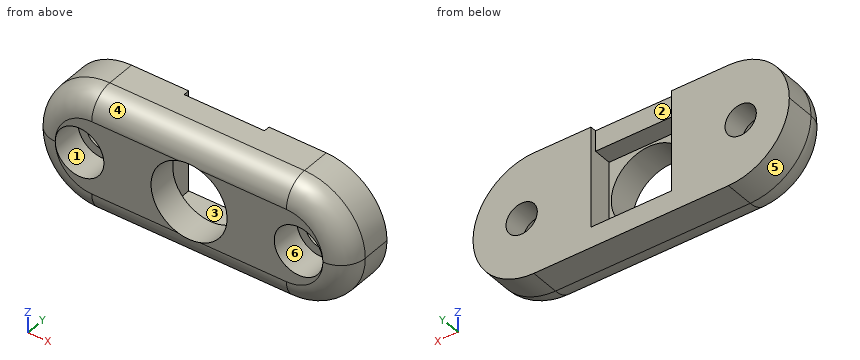
from build123d import *

# Parameters (mm, degrees)
SKETCH1_W                 = 33.02
SKETCH1_H                 = 12.7
SKETCH1_R                 = 3.96875
BOSS_EXTRUDE1_DEPTH       = 5.588
SKETCH2_W                 = 8.382
SKETCH2_H                 = 8.382
CUT_EXTRUDE1_DEPTH        = 2.54
F_4_CLEARANCE_HOLE1_D     = 3.2639
F_4_CLEARANCE_HOLE1_DEPTH = 12.7
F_4_CLEARANCE_HOLE1_TIP   = 0.980574487
FILLET1_R                 = 6.35
SKETCH7_W                 = 8.382
SKETCH7_H                 = 2.159
CUT_EXTRUDE2_DEPTH        = 0.635
SKETCH9_R                 = 2.54
CUT_EXTRUDE3_DEPTH        = 3.175
FILLET3_R                 = 2.54


# Some blends are built 0.0001 mm under size
with BuildPart() as part:
    # Sketch1 → Boss-Extrude1 (new body)
    with BuildSketch(Plane(origin=(0, 0, 0), x_dir=(1, 0, 0), z_dir=(0, 1, 0))):
        with Locations((-15.345948133, 4.349128799)):
            Rectangle(SKETCH1_W, SKETCH1_H)
        with Locations(Location((-15.345948133, 4.349128799, 0), (0, 0, 270))):
            Circle(SKETCH1_R, mode=Mode.SUBTRACT)
    extrude(amount=BOSS_EXTRUDE1_DEPTH)

    # Sketch2 → Cut-Extrude1 (cut)
    with BuildSketch(Plane(origin=(0, 5.588, 0), x_dir=(1, 0, 0), z_dir=(0, 1, 0))):
        with Locations((-15.345948133, 4.349128799)):
            Rectangle(SKETCH2_W, SKETCH2_H)
    extrude(amount=-CUT_EXTRUDE1_DEPTH, mode=Mode.SUBTRACT)

    # #4 Clearance Hole1
    with Locations(Plane(origin=(0, 0, 0), x_dir=(-1, 0, 0), z_dir=(0, -1, 0))):
        with Locations((3.915948133, 4.349128799), (26.775948133, 4.349128799)):
            Hole(F_4_CLEARANCE_HOLE1_D / 2, depth=F_4_CLEARANCE_HOLE1_DEPTH)
            with Locations((0, 0, -(F_4_CLEARANCE_HOLE1_DEPTH + F_4_CLEARANCE_HOLE1_TIP / 2))):  # 118° drill point
                Cone(0, F_4_CLEARANCE_HOLE1_D / 2, F_4_CLEARANCE_HOLE1_TIP, mode=Mode.SUBTRACT)

    # Fillet1
    fillet1_edges = [part.edges().sort_by_distance(p)[0] for p in [
        (-31.855948133, 2.794, 2.000871201),
        (-31.855948133, 2.794, -10.699128799),
        (1.164051867, 2.794, -10.699128799),
        (1.164051867, 2.794, 2.000871201),
    ]]
    fillet(fillet1_edges, radius=FILLET1_R - 0.0001)  # a hair under: the kernel refuses the full size

    # Sketch7 → Cut-Extrude2 (cut)
    with BuildSketch(Plane(origin=(0, 5.588, 0), x_dir=(1, 0, 0), z_dir=(0, 1, 0))):
        with Locations((-15.345948133, -0.921371201)):
            Rectangle(SKETCH7_W, SKETCH7_H)
    extrude(amount=-CUT_EXTRUDE2_DEPTH, mode=Mode.SUBTRACT)

    # Sketch9 → Cut-Extrude3 (cut)
    with BuildSketch(Plane.XZ):
        with Locations(Location((-3.915948133, -4.349128799, 0), (0, 0, 270))):
            Circle(SKETCH9_R)
        with Locations(Location((-26.775948133, -4.349128799, 0), (0, 0, 270))):
            Circle(SKETCH9_R)
    extrude(amount=-CUT_EXTRUDE3_DEPTH, mode=Mode.SUBTRACT)

    # Fillet3
    # the kernel refuses this fillet: 2.54 mm, written as the material it takes off along each edge
    with BuildSketch(Plane(origin=(-25.506048133, 0, 2.000871201), x_dir=(0, 0, -1), z_dir=(1, 0, 0))) as fillet3_piece_1:
        with BuildLine():
            CenterArc((FILLET3_R, FILLET3_R), FILLET3_R, 180, 90)
            Line((0, FILLET3_R), (0, 0))
            Line((0, 0), (FILLET3_R, 0))
        make_face()
    extrude(amount=20.3202, mode=Mode.SUBTRACT)
    with BuildSketch(Plane(origin=(-5.185848133, 0, -10.699128799), x_dir=(0, 1, 0), z_dir=(-1, 0, 0))) as fillet3_piece_2:
        with BuildLine():
            CenterArc((FILLET3_R, -FILLET3_R), FILLET3_R, 90, 90)
            Line((0, -FILLET3_R), (0, 0))
            Line((0, 0), (FILLET3_R, 0))
        make_face()
    extrude(amount=20.3202, mode=Mode.SUBTRACT)
    with BuildSketch(Plane(origin=(-5.185848133, 0, -4.349028799), x_dir=(1, 0, 0), z_dir=(0, 0, -1))) as fillet3_piece_3:
        with BuildLine():
            CenterArc((6.3499 - FILLET3_R, -FILLET3_R), FILLET3_R, 0, 90)
            Line((6.3499, -FILLET3_R), (6.3499, 0))
            Line((6.3499, 0), (6.3499 - FILLET3_R, 0))
        make_face()
    revolve(axis=Axis((-5.185848133, 0, -4.349028799), (0, -1, 0)), revolution_arc=90, mode=Mode.SUBTRACT)
    with BuildSketch(Plane(origin=(-5.185848133, 0, -4.349228799), x_dir=(0, 0, -1), z_dir=(-1, 0, 0))) as fillet3_piece_4:
        with BuildLine():
            CenterArc((6.3499 - FILLET3_R, -FILLET3_R), FILLET3_R, 0, 90)
            Line((6.3499, -FILLET3_R), (6.3499, 0))
            Line((6.3499, 0), (6.3499 - FILLET3_R, 0))
        make_face()
    revolve(axis=Axis((-5.185848133, 0, -4.349228799), (0, -1, 0)), revolution_arc=90, mode=Mode.SUBTRACT)
    with BuildSketch(Plane(origin=(-25.506048133, 0, -4.349228799), x_dir=(0, 0, -1), z_dir=(1, 0, 0))) as fillet3_piece_5:
        with BuildLine():
            CenterArc((6.3499 - FILLET3_R, FILLET3_R), FILLET3_R, 270, 90)
            Line((6.3499, FILLET3_R), (6.3499, 0))
            Line((6.3499, 0), (6.3499 - FILLET3_R, 0))
        make_face()
    revolve(axis=Axis((-25.506048133, 0, -4.349228799), (0, 1, 0)), revolution_arc=90, mode=Mode.SUBTRACT)
    with BuildSketch(Plane(origin=(-25.506048133, 0, -4.349028799), x_dir=(-1, 0, 0), z_dir=(0, 0, -1))) as fillet3_piece_6:
        with BuildLine():
            CenterArc((6.3499 - FILLET3_R, FILLET3_R), FILLET3_R, 270, 90)
            Line((6.3499, FILLET3_R), (6.3499, 0))
            Line((6.3499, 0), (6.3499 - FILLET3_R, 0))
        make_face()
    revolve(axis=Axis((-25.506048133, 0, -4.349028799), (0, 1, 0)), revolution_arc=90, mode=Mode.SUBTRACT)
    with BuildSketch(Plane(origin=(-31.855948133, 0, -4.349228799), x_dir=(1, 0, 0), z_dir=(0, 0, 1)), Plane(origin=(1.164051867, 0, -4.349028799), x_dir=(-1, 0, 0), z_dir=(0, 0, -1))) as fillet3_piece_7:
        with BuildLine():
            CenterArc((FILLET3_R, FILLET3_R), FILLET3_R, 180, 90)
            Line((0, FILLET3_R), (0, 0))
            Line((0, 0), (FILLET3_R, 0))
        make_face()
    extrude(amount=0.0002, mode=Mode.SUBTRACT)


solid = part.part
Geometry: final body of the model. Coordinates: model frame, mm. Face numbers are marked on the shaded views. A direction names the side the tool comes from. Round coordinates to 2 decimals unless told otherwise and drop trailing zeros. Write each loop counter-clockwise with the first axis right and the second up, starting at its lowest first coordinate (ties: lowest second). Pieces come first, ordered by that corner, then holes. Notation, with made-up numbers: M 86,-40 L 145,-40 A17 cw 145,-31 Z; hole C -26,40.25 d2. An arc over 180 degrees is marked long. Write item = value, one per line.
Item 1: Material intervals for line 1 along X through (y, z) = (5.05, -5.5); line 2 along X through (y, z) = (2.4, -5.25); line 3 along Z through (x, y) = (-26.5, 3.65), sorted ascending. Write a range as [from, to].
Findings:
line_1 = [-31.75, -27.93], [-25.62, -19.54], [-11.15, -5.07], [-2.76, 1.06]
line_2 = [-31.79, -29.15], [-24.4, -19.21], [-11.48, -6.29], [-1.54, 1.1]
line_3 = [-10.62, -5.96], [-2.74, 1.92]
Item 2: Access query for the marked faces 1, 2 and 3. Directions: +Z, -Z, +X, -X, +Y, -Y. A direction counts if a zero-diameter tool reaches every point of the face in a straight line with its end or side. Return the directions, or none.
Findings:
face_1 = -Y
face_2 = +Z, +Y
face_3 = +Y
Item 3: Section query B-B on x = -7.5. Return loops of the section in (y, z), then the cut area to 3 significant figures.
Findings:
outline = M 0,-8.16 A2.54 ccw 2.54,-10.7 L 5.59,-10.7 L 5.59,2 L 2.54,2 A2.54 ccw 0,-0.54 Z
area = 68.2 mm^2
Item 4: Pull-direction query (X, two-part tool) for the marked faces 4, 5 and 6; classes: pulls with the +X half, pulls with the -X half, needs draft (parallel to the pull), parting line crosses it, or undercut.
Findings:
face_4 = needs draft
face_5 = pulls with the -X half
face_6 = undercut
Item 5: Pin query (flat end, axial travel): P1, Ø2.5, axis at x = -27, z = -4, coming from the -Y side (3 decimals); P2, Ø2, axis at x = -3.92, z = -4.35, coming from the +Y side; P3, Ø1, axis at x = -13.5, z = 0.5, coming from the +Y side; P4, Ø2, axis at y = 4.5, z = -5.5, coming from the -X side. Return the tip coordinate at first contact, or that it passes through.
Findings:
P1 = 3.175
P2 = through
P3 = 4.95
P4 = -31.85
Item 6: Section query A-A on y = 4.55. State how many separate pieces and enclosed holes the cut face has, then the cut area to 3 significant figures.
Findings:
separate_pieces = 1
enclosed_holes = 3
area = 298 mm^2
